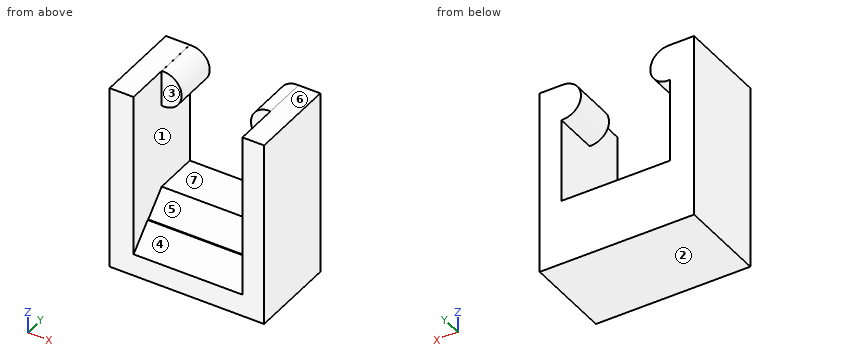
from build123d import *

# Parameters (mm, degrees)
F1_DEPTH    = 50.8
F2_R        = 10.405428205
F3_DEPTH    = 25.4
F4_T1_DEPTH = 62.2300039977
F5_W        = 88.3073359728
F5_H        = 50.8
F6_DEPTH    = 25.4
F7_SIZE     = 12.7


# Not quite as in the source:
# - a fillet or chamfer that OpenCascade refuses, or shapes differently, is made with other operations: its cross-section is extruded or revolved along the edge and cut away or added


with BuildPart() as f1:
    # F0 (on Front) → F1 (new body)
    with BuildSketch(Plane.XZ):
        Polygon((-31.2631689012, 40.7458357513), (-44.9346460508, 40.7458357513), (-44.9346460508, -40.4495000839), (43.372689922, -40.4495000839), (43.372689922, 40.7458357513), (30.9668350965, 40.7458357513), (30.9668350965, -28.2998345792), (-31.2631689012, -28.2998345792), align=None)
    extrude(amount=F1_DEPTH)

    # F2 (on Front) → F3 (join)
    with BuildSketch(Plane.XZ):
        with Locations((-30.2724801004, 30.3404075463)):
            Circle(F2_R)
        with Locations((30.2025526762, 30.3404075463)):
            Circle(F2_R)
    extrude(amount=F3_DEPTH)

    # F4: chamfer of 25.4 on 1 edges, made by hand

    # F4_s2 → F4_t1 (cut)
    with BuildSketch(Plane.YZ.offset(-31.2631689012)):
        Polygon((-50.8, -53.6998345792), (-25.4, -28.2998345792), (-50.8, -28.2998345792), align=None)
    extrude(amount=F4_T1_DEPTH, mode=Mode.SUBTRACT)

    # F5 (on face) → F6 (join)
    with BuildSketch(Plane(origin=(0, 0, -40.4495000839), x_dir=(1, 0, 0), z_dir=(0, 0, -1))):
        with Locations((-0.7809780644, 25.4)):
            Rectangle(F5_W, F5_H)
    extrude(amount=F6_DEPTH)

    # F7
    f7_edges = [f1.edges().sort_by_distance(p)[0] for p in [
        (-0.148167, -50.8, -40.4495),
    ]]
    chamfer(f7_edges, length=F7_SIZE)


solid = f1.part
Could you check a few things on this model? Use its own coordinates, in mm. Face numbers are marked on the shaded views. A direction names the side the tool comes from. Give positions to 0.01 mm unless a question says otherwise; leave off trailing zeros. Order: outer loops, then holes, each group sorted by start corner. A loop starts at its lowest first (then second) coordinate and runs counter-clockwise, first axis right, second up.
1. For pin 1 (9 mm diameter, centred on x = -23, z = 29.5, fed in from -Y); pin 2 (8 mm diameter, centred on x = 4.5, y = -32.5, fed in from +Z), each with a flat end and sliding along its axis, tell me the tip position at first contact or that it passes through.
Answers below:
pin 1: stops at y = -25.4
pin 2: stops at z = -31.4
2. Suppose I cut it at D-D (x = -9.5). Write out the boundary of the cut face in (y, z).
Answers below:
outline: (-50.8, -65.85) - (0, -65.85) - (0, -28.3) - (-25.4, -28.3) - (-37.55, -40.45) - (-38.1, -40.45) - (-50.8, -53.15) - close
3. Suppose I cut it at B-B (x = -22). Write out the boundary of the cut face in (y, z).
Answers below:
outline: (-50.8, -65.85) - (0, -65.85) - (0, -28.3) - (-25.4, -28.3) - (-37.55, -40.45) - (-38.1, -40.45) - (-50.8, -53.15) - close; (-25.4, 24.03) - (0, 24.03) - (0, 36.65) - (-25.4, 36.65) - close
4. Thinking about a two-plate mould opening in Z: for the marked faces 1, 2, 3 and 4, which applies, +Z half, -Z half, draft (parallel to the pull), parting line (faces both ways), or undercut?
Answers below:
face 1: undercut
face 2: -Z half
face 3: draft
face 4: +Z half
5. Which directions (+Z, -Z, +X, -X, +Y, -Y) give clear straight access to the entire face, cutting with the end or side of a thin tool? Please do the marked faces 5, 6 and 7.
Answers below:
face 5: +Z, -Y
face 6: +Z, +X, -X, +Y, -Y
face 7: +Y, -Y
6. I need wall thicknesses on L1, parallel to X at y = -45, z = -28.5; L2, parallel to Z at x = 9.5, y = -23; L3, parallel to X at y = -13, z = 23.5. Which ranges of each line are inside material? Lowest first, please.
Answers below:
L1: x = -44.93 to -31.26, 30.97 to 43.37
L2: z = -65.85 to -28.3
L3: x = -44.93 to -22.43, 22.36 to 43.37
7. Suppose I cut it at A-A (z = -25.5). Write out the boundary of the cut face in (x, y).
Answers below:
outline: (-44.93, -50.8) - (-31.26, -50.8) - (-31.26, 0) - (-44.93, 0) - close; (30.97, -50.8) - (43.37, -50.8) - (43.37, 0) - (30.97, 0) - close
